Geometry check sheet. Reference: the model listing, model coordinates, mm. A direction names the side the tool comes from. Give positions to 0.01 mm unless a question says otherwise; leave off trailing zeros. Loops run counter-clockwise (first coordinate to the right, second up) from the corner with the lowest first, then second, coordinate; pieces in that order, holes last. Notation, with made-up numbers: (61.25, 66.5) - (66.25, 66.5) arc R19 cw to (66.25, 82.5) - close; hole circle Ø5 at (16.25, 20.25). An arc over 180 degrees is marked (long way). Use a Markdown table: item, result. Add a question column.
1. Cross-section at A-A on x = -21. Enter the section's corners in (y, z), and give its area (3 significant figures).
2. Depth check by flat-ended pin: P1, Ø14.5, axis at x = -3, y = -6, coming from the +Z side; P2, Ø8, axis at x = -63.5, y = -22.5, coming from the +Z side. Enter the tip coordinate at first touch or a pass-through.
3. Set-up check for faces 5 (the flat face through (-1, 0, 0)), 6 (the flat face through (53, 0, 5)): record each of +Z, -Z, +X, -X, +Y, -Y from which the full face is reachable in a straight line by a thin tool's end or side.
4. Cross-section at B-B on z = 11. Count the separate pieces of the cut face and the enclosed holes in it, and give its area (3 significant figures).
5. Material ranges on L1, parallel to X at y = -11, z = 25; L2, parallel to Y at x = 56.5, z = 42; L3, parallel to Z at x = -49, y = 7, recorded low to high.
6. Draft check along X on faces 1 (the flat face through (81, 0, 24)), 2 (the flat face through (0, 27, 28)), 3 (the flat face through (-1, -30, 24)), 4 (the flat face through (-81, 0, 24)). Enter one of: pulls with the +X half, pulls with the -X half, needs draft (parallel to the pull), parting line crosses it, or undercut.
from build123d import *

# Parameters (mm, degrees)
SKETCH1_W           = 162
SKETCH1_H           = 60
BOSS_EXTRUDE1_DEPTH = 50
SKETCH2_W           = 50
SKETCH2_H           = 54
CUT_EXTRUDE1_DEPTH  = 45
FILLET1_R           = 1


with BuildPart() as part:
    # Sketch1 → Boss-Extrude1 (new body)
    with BuildSketch(Plane.XY):
        Rectangle(SKETCH1_W, SKETCH1_H)
    extrude(amount=BOSS_EXTRUDE1_DEPTH)

    # Sketch2 → Cut-Extrude1 (cut)
    with BuildSketch(Plane.XY.offset(50)):
        with Locations((-53, 0)):
            Rectangle(SKETCH2_W, SKETCH2_H)
        Rectangle(SKETCH2_W, SKETCH2_H)
        with Locations((53, 0)):
            Rectangle(SKETCH2_W, SKETCH2_H)
    extrude(amount=-CUT_EXTRUDE1_DEPTH, mode=Mode.SUBTRACT)

    # Fillet1
    fillet1_edges = [part.edges().sort_by_distance(p)[0] for p in [
        (81, 0, 50),
        (0, 30, 50),
        (-78, 0, 5),
        (-78, -27, 27.5),
        (-53, 27, 5),
        (-78, 27, 27.5),
        (-28, 0, 5),
        (-28, 27, 27.5),
        (-53, -27, 5),
        (-28, -27, 27.5),
        (-78, 0, 50),
        (-53, -27, 50),
        (-28, 0, 50),
        (-53, 27, 50),
        (-25, 0, 5),
        (-25, -27, 27.5),
        (0, 27, 5),
        (-25, 27, 27.5),
        (25, 0, 5),
        (25, 27, 27.5),
        (0, -27, 5),
        (25, -27, 27.5),
        (-25, 0, 50),
        (0, -27, 50),
        (25, 0, 50),
        (0, 27, 50),
        (28, 0, 5),
        (28, -27, 27.5),
        (53, 27, 5),
        (28, 27, 27.5),
        (78, 0, 5),
        (78, 27, 27.5),
        (53, -27, 5),
        (28, 0, 50),
        (53, -27, 50),
        (78, 0, 50),
        (53, 27, 50),
        (-81, 0, 50),
        (-81, 30, 25),
        (81, 30, 25),
        (81, -30, 25),
        (-81, -30, 25),
        (0, -30, 50),
    ]]
    fillet(fillet1_edges, radius=FILLET1_R)


solid = part.part
Values found:
| question | item | result |
|---|---|---|
| 1 | outline | (-30, 0) - (30, 0) - (30, 49) arc R1 ccw to (29, 50) - (28, 50) arc R1 ccw to (27, 49) - (27, 6) arc R1 cw to (26, 5) - (-26, 5) arc R1 cw to (-27, 6) - (-27, 49) arc R1 ccw to (-28, 50) - (-29, 50) arc R1 ccw to (-30, 49) - close |
| 1 | area | 570 mm2 |
| 2 | P1 | stops at z = 5 |
| 2 | P2 | stops at z = 5.13 |
| 3 | face 5 | -Z, +X, -X, +Y, -Y |
| 3 | face 6 | +Z |
| 4 | separate pieces | 1 |
| 4 | enclosed holes | 3 |
| 4 | area | 1,620 mm2 |
| 5 | L1 | x = -81 to -78, -28 to -25, 25 to 28, 78 to 81 |
| 5 | L2 | y = -30 to -27, 27 to 30 |
| 5 | L3 | z = 0 to 5 |
| 6 | face 1 | pulls with the +X half |
| 6 | face 2 | undercut |
| 6 | face 3 | needs draft |
| 6 | face 4 | pulls with the -X half |
